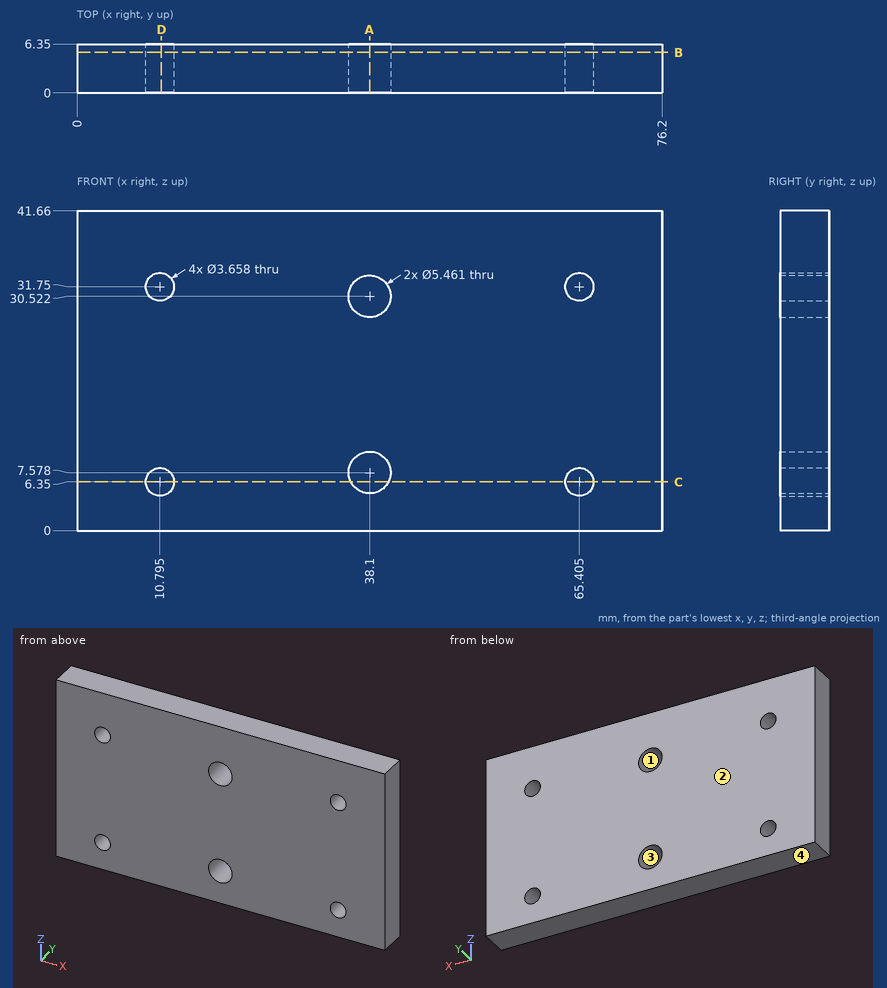
Job drawing, mm, ordinate dimensions from the low corner. One solid piece. Give positions to 0.01 mm unless a question says otherwise; leave off trailing zeros. Loops run counter-clockwise (first coordinate to the right, second up) from the corner with the lowest first, then second, coordinate; pieces in that order, holes last. Notation, with made-up numbers: (43.5, 32.5) -> (97.5, 32.5) arc R24 ccw to (97.5, 44.5) -> close; hole circle Ø1 at (62, 71.25). An arc over 180 degrees is marked (long way). Write each question's results on one line, items separated by ' | '. Start each with the question number.
Q1. Pin check, flat tip, straight feed: P1, Ø5, axis at x = 10.795, z = 31.75, coming from the -Y side. Stop position of the tip, or through.
Q2. Band-saw the part on B-B on y = 5.25. Count the separate pieces of the cut face and the enclosed holes in it, plus the area to 3 significant figures.
Q3. Band-saw the part on D-D on x = 11. List the corners of the cut face in (y, z), plus the area to 3 significant figures.
Q4. Pull direction Z, two halves, no side cores. Call the marked faces 1, 2, 3 and 4: +Z half, -Z half, draft (parallel to the pull), parting line (faces both ways), or undercut.
Q5. Band-saw the part on A-A on x = 38.1. List the corners of the cut face in (y, z).
Q6. Wall check: L1, parallel to Z at x = 38.1, y = 3; L2, parallel to X at y = 2.5, z = 7 (1 decimal); L3, parallel to X at y = 4.75, z = 31.75 (1 decimal). Give the ranges that are in metal, low to high.
Q7. Band-saw the part on C-C on z = 6.35. List the corners of the cut face in (x, y).
Results are:
1) P1: stops at y = 0
2) separate pieces: 1 | enclosed holes: 6 | area: 3,090 mm²
3) outline: (0, 0) -> (6.35, 0) -> (6.35, 4.53) -> (0, 4.53) -> close; (0, 8.17) -> (6.35, 8.17) -> (6.35, 29.93) -> (0, 29.93) -> close; (0, 33.57) -> (6.35, 33.57) -> (6.35, 41.66) -> (0, 41.66) -> close | area: 218 mm²
4) face 1: undercut | face 2: draft | face 3: undercut | face 4: -Z half
5) outline: (0, 0) -> (6.35, 0) -> (6.35, 4.85) -> (0, 4.85) -> close; (0, 10.31) -> (6.35, 10.31) -> (6.35, 27.79) -> (0, 27.79) -> close; (0, 33.25) -> (6.35, 33.25) -> (6.35, 41.66) -> (0, 41.66) -> close
6) L1: z = 0 to 4.85, 10.31 to 27.79, 33.25 to 41.66 | L2: x = 0 to 9.1, 12.5 to 35.4, 40.8 to 63.7, 67.1 to 76.2 | L3: x = 0 to 9, 12.6 to 35.7, 40.5 to 63.6, 67.2 to 76.2
7) outline: (0, 0) -> (8.97, 0) -> (8.97, 6.35) -> (0, 6.35) -> close; (12.62, 0) -> (35.66, 0) -> (35.66, 6.35) -> (12.62, 6.35) -> close; (40.54, 0) -> (63.58, 0) -> (63.58, 6.35) -> (40.54, 6.35) -> close; (67.23, 0) -> (76.2, 0) -> (76.2, 6.35) -> (67.23, 6.35) -> close
